```python
from build123d import *

# Parameters (mm, degrees)
ESQUISSE1_W                = 15
ESQUISSE1_H                = 2.5
EXTRUSION1_DEPTH           = 50
ESQUISSE2_R                = 1.5
EXTRUSION2_DEPTH           = 51.621141828
R_P_TITION_LIN_AIRE1_COUNT = 2
R_P_TITION_LIN_AIRE1_PITCH = 15
CONG_1_R                   = 7.5
ESQUISSE5_R                = 1.05
ENL_V_MAT_EXTRU_3_DEPTH    = 10
ESQUISSE6_R                = 1.05
ENL_V_MAT_EXTRU_4_DEPTH    = 10


with BuildPart() as part:
    # Esquisse1 → Extrusion1 (new body)
    with BuildSketch(Plane.XY):
        Rectangle(ESQUISSE1_W, ESQUISSE1_H)
    extrude(amount=EXTRUSION1_DEPTH)

    # Esquisse2 → Extrusion2 (cut, through all)
    with BuildSketch(Plane(origin=(0, 1.25, 0), x_dir=(1, 0, 0), z_dir=(0, 1, 0))):
        with Locations(Location((0, -45, 0), (0, 0, 270))):
            Circle(ESQUISSE2_R)
    extrusion2 = extrude(amount=-EXTRUSION2_DEPTH, mode=Mode.SUBTRACT)

    # Répétition linéaire1: Extrusion2 ×2
    with Locations(*[(0, 0, -i * R_P_TITION_LIN_AIRE1_PITCH) for i in range(1, R_P_TITION_LIN_AIRE1_COUNT)]):
        add(extrusion2, mode=Mode.SUBTRACT)

    # Congé1
    cong_1_edges = [part.edges().sort_by_distance(p)[0] for p in [
        (-7.5, 0, 50),
        (7.5, 0, 50),
    ]]
    fillet(cong_1_edges, radius=CONG_1_R - 0.0001)  # a hair under: the kernel refuses the full size

    # Esquisse5 → Enlèv. mat.-Extru.3 (cut)
    with BuildSketch(Plane(origin=(0, 1.25, 0), x_dir=(-1, 0, 0), z_dir=(0, 1, 0))):
        with Locations(Location((0, 6.249569422, 0), (0, 0, 90))):
            Circle(ESQUISSE5_R)
    extrude(amount=-ENL_V_MAT_EXTRU_3_DEPTH, mode=Mode.SUBTRACT)

    # Esquisse6 → Enlèv. mat.-Extru.4 (cut)
    with BuildSketch(Plane(origin=(0, 1.25, 0), x_dir=(1, 0, 0), z_dir=(0, 1, 0))):
        with Locations(Location((0, -15.849569422, 0), (0, 0, 270))):
            Circle(ESQUISSE6_R)
    extrude(amount=-ENL_V_MAT_EXTRU_4_DEPTH, mode=Mode.SUBTRACT)


solid = part.part
```
Source: CAD feature listing. Evaluate the final solid. Frame: model axes, mm. Give positions to 0.01 mm unless a question says otherwise; leave off trailing zeros. Loops run counter-clockwise (first coordinate to the right, second up) from the corner with the lowest first, then second, coordinate; pieces in that order, holes last. Notation, with made-up numbers: (54, 7) -> (90, 7) arc R18 ccw to (90, 12) -> close; hole circle Ø2 at (89, -36). An arc over 180 degrees is marked (long way). Put each result on its own line as item: value. Start each with the question number.
1) Cut plane C-C (z = 45). Return loops of the section in (x, y), then the cut area to 3 significant figures.
2) Cut plane A-A (z = 30). Return loops of the section in (x, y).
3) Cut plane B-B (y = 0.3). State how many separate pieces and enclosed holes the cut face has, then the cut area to 3 significant figures.
4) Contact query for a flat-ended pin moving along its axis: P1, Ø1.9, axis at x = 0, z = 6.25, coming from the -Y side. Output: stop coordinate, or through.
5) Draft query along X for faces 1 (the face through (7.5, 0, 21)), 2 (the face through (0, -1.25, 25)), 3 (the face through (-5.361, 0.018, 47.745)), 4 (the face through (0.07, 0.02, 43.5)). Return one class per face: released by +X, released by -X, zero draft, split by the parting line, or undercut.
6) Cut plane D-D (x = 5). Return loops of the section in (y, z).
7) Material intervals for probe 1 along Z at (x, y) = (-0.25, 0.15); probe 2 along X at (y, z) = (0.5, 30); probe 3 along X at (y, z) = (0.05, 45.5), sorted ascending.
Results are:
1. outline: (-7.07, -1.25) -> (-1.5, -1.25) -> (-1.5, 1.25) -> (-7.07, 1.25) -> close; (1.5, -1.25) -> (7.07, -1.25) -> (7.07, 1.25) -> (1.5, 1.25) -> close
1. area: 27.9 mm2
2. outline: (-7.5, -1.25) -> (-1.5, -1.25) -> (-1.5, 1.25) -> (-7.5, 1.25) -> close; (1.5, -1.25) -> (7.5, -1.25) -> (7.5, 1.25) -> (1.5, 1.25) -> close
3. separate pieces: 1
3. enclosed holes: 4
3. area: 705 mm2
4. P1: passes through
5. face 1: released by +X
5. face 2: zero draft
5. face 3: released by -X
5. face 4: undercut
6. outline: (-1.25, 0) -> (1.25, 0) -> (1.25, 48.09) -> (-1.25, 48.09) -> close
7. probe 1: z = 0 to 5.23, 7.27 to 14.83, 16.87 to 28.52, 31.48 to 43.52, 46.48 to 50
7. probe 2: x = -7.5 to -1.5, 1.5 to 7.5
7. probe 3: x = -6.87 to -1.41, 1.41 to 6.87
